Design review of the part built by this model. Coordinates are the model's own, in mm. Coordinates: 2 decimals unless noted, no trailing zeros. Loops run counter-clockwise (first coordinate to the right, second up) from the corner with the lowest first, then second, coordinate; pieces in that order, holes last. Notation, with made-up numbers: (19.5, 80.5) -> (55.5, 80.5) arc R20 ccw to (55.5, 86.5) -> close; hole circle Ø2 at (-23, 42.25). An arc over 180 degrees is marked (long way). Use a Markdown table: item, result. Add a question column.
Q1. Take a section at C-C on z = 37.5. Write out the cut boundary in (x, y) (1 decimal).
Q2. Take a section at B-B on x = 0. Write out the cut boundary in (y, z) (1 decimal), plus the area to 3 significant figures.
Q3. Clearance check with flat-ended pins moving along their axes: pin 1 Ø2.5 at (x, z) = (-0.5, 94) entering from +Y; pin 2 Ø1 at (x, z) = (-1.5, -88) entering from +Y. State where each tip first meets the part, or that it passes through.
Q4. For probe 1 along Z at (x, y) = (-2.25, 3); probe 2 along X at (y, z) = (-0.5, -103.5); probe 3 along Y at (x, z) = (0.25, -45.5), list the stretches that pass through material, from the lowest coordinate up.
Q5. Take a section at D-D on z = 89. Write out the cut boundary in (x, y), plus the area to 3 significant figures.
Q6. Take a section at A-A on y = 0. Write out the cut boundary in (x, z) (1 decimal).
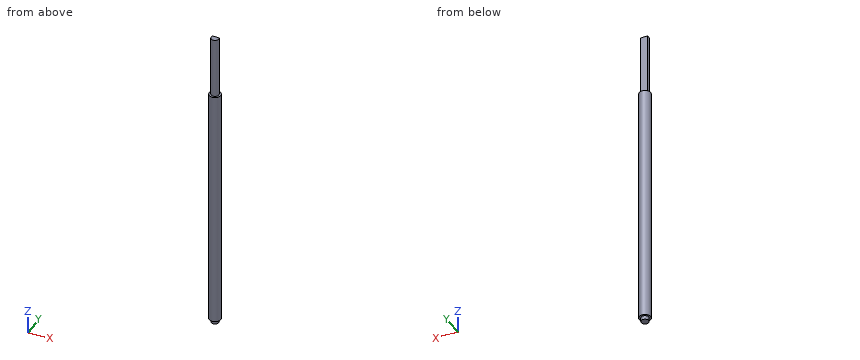
Autodesk Inventor part; units mm, degrees
ref_plane "YZ Plane" through (0, 0, 0) normal (1, 0, 0) x (0, 1, 0)
ref_plane "XZ Plane" through (0, 0, 0) normal (0, 1, 0) x (-1, 0, 0)
ref_plane "XY Plane" through (0, 0, 0) normal (0, 0, 1) x (1, 0, 0)
sketch "Sketch1" plane through (0, 0, 0) normal (0, 0, 1) x (1, 0, 0)
  circle A0 centre (0, 0) radius 4.7625
  dimension "d0" = 9.525
extrude "Extrusion1" add sketch "Sketch1" along normal mid plane 254
thread "Thread1"
sketch "Sketch2" plane through (0, 0, 127) normal (0, 0, 1) x (1, 0, 0)
  arc A0 (-2.7496, 1.5875) -> (2.7496, 1.5875) centre (0, 0) ccw
  line L0 (-2.7496, 1.5875) -> (2.7496, 1.5875)
  circle A1 centre (0, 0) radius 8.1081
  dimension "d5" = 6.35
  dimension "d6" = 1.5875
extrude "Extrusion2" cut sketch "Sketch2" against normal blind 50.8
sketch "Sketch4" plane through (0, 0, -127) normal (0, 0, -1) x (-1, 0, 0)
  circle A0 centre (0, 0) radius 3.175
  dimension "d16" = 6.35
extrude "Extrusion3" add sketch "Sketch4" along normal blind 3.175
Answer list:
| question | item | result |
|---|---|---|
| 1 | outline | circle Ø9.5 at (0, 0) |
| 2 | outline | (-4.8, -127) -> (-3.2, -127) -> (-3.2, -130.2) -> (3.2, -130.2) -> (3.2, -127) -> (4.8, -127) -> (4.8, 76.2) -> (1.6, 76.2) -> (1.6, 127) -> (-3.2, 127) -> (-3.2, 76.2) -> (-4.8, 76.2) -> close |
| 2 | area | 2,200 mm² |
| 3 | pin 1 | y = 1.59 |
| 3 | pin 2 | y = 4.66 |
| 4 | probe 1 | -127 to 76.2 |
| 4 | probe 2 | -4.74 to 4.74 |
| 4 | probe 3 | -4.76 to 4.76 |
| 5 | outline | (-2.75, 1.59) arc R3.17 ccw (long way) to (2.75, 1.59) -> close |
| 5 | area | 25.5 mm² |
| 6 | outline | (-4.8, -127) -> (-3.2, -127) -> (-3.2, -130.2) -> (3.2, -130.2) -> (3.2, -127) -> (4.8, -127) -> (4.8, 76.2) -> (3.2, 76.2) -> (3.2, 127) -> (-3.2, 127) -> (-3.2, 76.2) -> (-4.8, 76.2) -> close |
